Read the model definition and answer for the solid it produces. Units are mm, in the model's axes. Face numbers are marked on the shaded views. A direction names the side the tool comes from. Coordinates: 2 decimals unless noted, no trailing zeros. Write each loop counter-clockwise with the first axis right and the second up, starting at its lowest first coordinate (ties: lowest second). Pieces come first, ordered by that corner, then holes.
(1) Section A-A on y = 0.25 is taken. Write down the section's boundary in (x, z).
(2) Find the intervals of material crossed by probe 1 along Y at (x, z) = (11, -12.25); probe 2 along X at (y, z) = (0.5, -13); probe 3 along X at (y, z) = (-3.5, -0.5), in increasing order.
(3) Which of the six approach directions +Z, -Z, +X, -X, +Y, -Y give full straight-line access (tool end or side, diameter ignored) to the marked faces 1, 2, 3 and 4?
(4) Section C-C on x = -0.5 is taken. Write down the section's boundary in (y, z), then the cut area to 3 significant figures.
(5) Given pin 1 (4 mm diameter, centred on y = -2, z = -7, fed in from -X); pin 2 (4.5 mm diameter, centred on x = 0, z = -7, fed in from -Y); pin 3 (5 mm diameter, centred on x = 0.5, z = -7.5, fed in from +Y), each flat-ended and moving along its own axis, determine where each tip first touches the part or whether it passes through.
(6) Section D-D on y = -3.5 is taken. Write down the section's boundary in (x, z), then the cut area to 3 significant figures.
(7) Section B-B on z = 0.5 is taken. Write down the section's boundary in (x, y).
(8) The mould has two halves that part along Y. Classify the marked faces 5, 6 and 7: +Y half, -Y half, draft (parallel to the pull), parting line (faces both ways), or undercut.
from build123d import *

# Parameters (mm, degrees)
F0_W     = 40
F0_H     = 10
F0_W_2   = 36
F0_H_2   = 6
F1_DEPTH = 15
F2_W     = 42
F2_H     = 12
F2_W_2   = 40
F2_H_2   = 10
F2_W_3   = 36
F2_H_3   = 6
F3_DEPTH = 2
F4_R     = 1


with BuildPart() as f1:
    # F0 (on Top) → F1 (new body)
    with BuildSketch(Plane.XY):
        Rectangle(F0_W, F0_H)
        Rectangle(F0_W_2, F0_H_2, mode=Mode.SUBTRACT)
    extrude(amount=-F1_DEPTH)

    # F2 (on face) → F3 (join)
    with BuildSketch(Plane.XY):
        Rectangle(F2_W, F2_H)
        Rectangle(F2_W_2, F2_H_2, mode=Mode.SUBTRACT)
        Rectangle(F2_W_2, F2_H_2)
        Rectangle(F2_W_3, F2_H_3, mode=Mode.SUBTRACT)
    extrude(amount=F3_DEPTH)

    # F4
    f4_edges = [f1.edges().sort_by_distance(p)[0] for p in [
        (21, 6, 1),
        (21, -6, 1),
        (-21, 6, 1),
        (-21, -6, 1),
        (20, 5, -7.5),
        (20, -5, -7.5),
        (-20, -5, -7.5),
        (-20, 5, -7.5),
        (18, 3, -6.5),
        (-18, 3, -6.5),
        (-18, -3, -6.5),
        (18, -3, -6.5),
    ]]
    fillet(f4_edges, radius=F4_R)


solid = f1.part
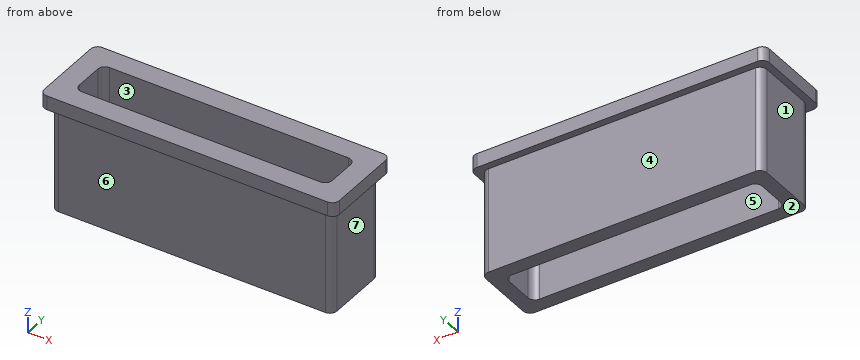
Response:
1. outline: (-21, 0) - (-20, 0) - (-20, -15) - (-18, -15) - (-18, 2) - (-21, 2) - close; (18, -15) - (20, -15) - (20, 0) - (21, 0) - (21, 2) - (18, 2) - close
2. probe 1: y = -5 to -3, 3 to 5
2. probe 2: x = -20 to -18, 18 to 20
2. probe 3: x = -20 to 20
3. face 1: -Z, -X, +Y, -Y
3. face 2: -Z, +X, -X, +Y, -Y
3. face 3: +Z, -Z
3. face 4: -Z, +X, -X, +Y
4. outline: (-6, 0) - (-5, 0) - (-5, -15) - (-3, -15) - (-3, 2) - (-6, 2) - close; (3, -15) - (5, -15) - (5, 0) - (6, 0) - (6, 2) - (3, 2) - close
4. area: 72.0 mm2
5. pin 1: stops at x = -20
5. pin 2: stops at y = -5
5. pin 3: stops at y = 5
6. outline: (-21, 0) - (-20, 0) - (-20, -15) - (20, -15) - (20, 0) - (21, 0) - (21, 2) - (-21, 2) - close
6. area: 684 mm2
7. outline: (-21, -5) arc R1 ccw to (-20, -6) - (20, -6) arc R1 ccw to (21, -5) - (21, 5) arc R1 ccw to (20, 6) - (-20, 6) arc R1 ccw to (-21, 5) - close; hole (-18, -2) arc R1 ccw to (-17, -3) - (17, -3) arc R1 ccw to (18, -2) - (18, 2) arc R1 ccw to (17, 3) - (-17, 3) arc R1 ccw to (-18, 2) - close
8. face 5: undercut
8. face 6: -Y half
8. face 7: draft
